```python
from build123d import *

# Parameters (mm, degrees)
BOSS_EXTRUDE1_DEPTH            = 7.5
BOSS_EXTRUDE2_DEPTH            = 7.5
CUT_EXTRUDE1_DEPTH             = 5
F_3_2_3_2_DIAMETER_HOLE1_D     = 3.2
FILLET1_R                      = 2
FILLET2_R                      = 2
CUT_EXTRUDE2_REACH             = 39.378
CUT_EXTRUDE2_END_RADIUS        = 224.5
SKETCH22_R                     = 2.1
CUT_EXTRUDE2_DIRECTION_2_DEPTH = 0.9
SKETCH23_R                     = 3.5
CUT_EXTRUDE3_DEPTH             = 2.6
SKETCH24_W                     = 2.6
SKETCH24_H                     = 3.5


with BuildPart() as part:
    # Sketch1 → Boss-Extrude1 (new body)
    with BuildSketch(Plane(origin=(0, 0, 0), x_dir=(1, 0, 0), z_dir=(0, 1, 0))):
        with BuildLine():
            ThreePointArc((-207.414551525, 32.851237658), (-210, 0), (-207.414551525, -32.851237658))
            Line((-207.414551525, -32.851237658), (-217.291434931, -34.415582309))
            ThreePointArc((-217.291434931, -34.415582309), (-220, 0), (-217.291434931, 34.415582309))
            Line((-217.291434931, 34.415582309), (-207.414551525, 32.851237658))
        make_face()
        with BuildLine():
            ThreePointArc((-217.291434931, -34.415582309), (-220, 0), (-217.291434931, 34.415582309))
            Line((-217.291434931, 34.415582309), (-220.254499953, 34.884885704))
            ThreePointArc((-220.254499953, 34.884885704), (-223, 0), (-220.254499953, -34.884885704))
            Line((-220.254499953, -34.884885704), (-217.291434931, -34.415582309))
        make_face()
        with BuildLine():
            Line((-202.969953992, 32.147282566), (-207.414551525, 32.851237658))
            ThreePointArc((-207.414551525, 32.851237658), (-210, 0), (-207.414551525, -32.851237658))
            Line((-207.414551525, -32.851237658), (-202.969953992, -32.147282566))
            ThreePointArc((-202.969953992, -32.147282566), (-205.5, 0), (-202.969953992, 32.147282566))
        make_face()
    extrude(amount=BOSS_EXTRUDE1_DEPTH)

    # Sketch19 → Boss-Extrude2 (add)
    with BuildSketch(Plane(origin=(0, 0, 0), x_dir=(1, 0, 0), z_dir=(0, 1, 0))):
        with BuildLine():
            Line((-224.019328267, 14.683002512), (-222.522539882, 14.584897818))
            ThreePointArc((-222.522539882, 14.584897818), (-223, 0), (-222.522539882, -14.584897818))
            Line((-222.522539882, -14.584897818), (-224.019328267, -14.683002512))
            ThreePointArc((-224.019328267, -14.683002512), (-224.5, 0), (-224.019328267, 14.683002512))
        make_face()
    extrude(amount=BOSS_EXTRUDE2_DEPTH)

    # Sketch15 → Cut-Extrude1 (cut)
    with BuildSketch(Plane(origin=(0, 7.5, 0), x_dir=(1, 0, 0), z_dir=(0, 1, 0))):
        with BuildLine():
            Line((-219.772609758, 10), (-209.761769634, 10))
            ThreePointArc((-209.761769634, 10), (-208.900850883, 21.457737542), (-207.414551525, 32.851237658))
            Line((-207.414551525, 32.851237658), (-217.291434931, 34.415582309))
            ThreePointArc((-217.291434931, 34.415582309), (-218.872736893, 22.242415451), (-219.772609758, 10))
        make_face()
        with BuildLine():
            ThreePointArc((-207.414551525, -32.851237658), (-208.900850883, -21.457737542), (-209.761769634, -10))
            Line((-209.761769634, -10), (-219.772609758, -10))
            ThreePointArc((-219.772609758, -10), (-218.872736893, -22.242415451), (-217.291434931, -34.415582309))
            Line((-217.291434931, -34.415582309), (-207.414551525, -32.851237658))
        make_face()
    extrude(amount=-CUT_EXTRUDE1_DEPTH, mode=Mode.SUBTRACT)

    # Ø3.2 (3.2) Diameter Hole1 (through all)
    with Locations(Plane(origin=(0, 0, 0), x_dir=(-1, 0, 0), z_dir=(0, -1, 0))):
        with Locations((214.18186009, -18.738484691), (214.18186009, 18.738484691)):
            Hole(F_3_2_3_2_DIAMETER_HOLE1_D / 2)

    # Fillet1
    fillet1_edges = [part.edges().sort_by_distance(p)[0] for p in [
        (-220.254499953, 3.75, 34.884885704),
        (-220.254499953, 3.75, -34.884885704),
        (-202.969953992, 3.75, -32.147282566),
        (-202.969953992, 3.75, 32.147282566),
    ]]
    fillet(fillet1_edges, radius=FILLET1_R)

    # Fillet2
    # the kernel refuses this fillet: 2 mm, written as the material it adds along each edge
    with BuildSketch(Plane(origin=(-222.522539882, 0, -14.584897818), x_dir=(0.06970140258603677, 0, -0.9975678996827931), z_dir=(0, 1, 0))) as fillet2_piece_1:
        with BuildLine():
            CenterArc((1.930030715, 1.99998144), FILLET2_R, 194.477374901, 75.275788142)
            Line((-0.006462156, 1.49998608), (-0.045192014, 1.489986173))
            ThreePointArc((-0.045192014, 1.489986173), (-0.043230707, 0.749820716), (-0.039999629, -0.000172324))
            Line((-0.039999629, -0.000172324), (0.000172324, -0.039999629))
            ThreePointArc((0.000172324, -0.039999629), (0.960707253, -0.037930577), (1.921242182, -0.039999629))
            Line((1.921242182, -0.039999629), (1.921414506, 0))
        make_face()
    extrude(amount=7.5)
    with BuildSketch(Plane(origin=(-222.522539882, 0, 14.584897818), x_dir=(-0.9978589232386029, 0, 0.06540312923015226), z_dir=(0, 1, 0))) as fillet2_piece_2:
        with BuildLine():
            CenterArc((1.991648107, 1.938628933), FILLET2_R, 180.493673912, 75.275788142)
            Line((-0.008277654, 1.921396676), (-0.048276169, 1.92105203))
            ThreePointArc((-0.048276169, 1.92105203), (-0.042069052, 0.960534929), (-0.04, 0))
            Line((-0.04, 0), (0, -0.04))
            ThreePointArc((0, -0.04), (0.75, -0.04), (1.490167038, -0.038772579))
            Line((1.490167038, -0.038772579), (1.5, 0))
        make_face()
    extrude(amount=7.5)

    # Cut-Extrude2: up to this cylinder (the profile starts inside it)
    cut_extrude2_end = Plane(origin=(0, 7.5, 0), z_dir=(0, -1, 0)) * Cylinder(CUT_EXTRUDE2_END_RADIUS, 528.756, mode=Mode.PRIVATE)
    # Sketch22 → Cut-Extrude2 (cut, up to the surface)
    with BuildSketch(Plane(origin=(-212.5, 0, 0), x_dir=(0, 0, -1), z_dir=(1, 0, 0)), mode=Mode.PRIVATE) as cut_extrude2_sk1:
        with Locations((0, 7.5)):
            Circle(SKETCH22_R)
    cut_extrude2_tool1 = extrude(cut_extrude2_sk1.sketch, amount=-CUT_EXTRUDE2_REACH, mode=Mode.PRIVATE) & cut_extrude2_end
    add(cut_extrude2_tool1.solids().sort_by_distance((-212.5, 7.5, 0))[0], mode=Mode.SUBTRACT)

    # Sketch22 → Cut-Extrude2 direction 2 (cut)
    with BuildSketch(Plane(origin=(-212.5, 0, 0), x_dir=(0, 0, -1), z_dir=(1, 0, 0))):
        with Locations((0, 7.5)):
            Circle(SKETCH22_R)
    extrude(amount=CUT_EXTRUDE2_DIRECTION_2_DEPTH, mode=Mode.SUBTRACT)

    # Sketch23 → Cut-Extrude3 (cut)
    with BuildSketch(Plane.ZY.offset(211.6)):
        with Locations((0, 7.439199918)):
            Circle(SKETCH23_R)
    extrude(amount=CUT_EXTRUDE3_DEPTH, mode=Mode.SUBTRACT)

    # Sketch24 → Cut-Revolve1 (revolve, cut)
    with BuildSketch(Plane(origin=(0, 7.5, 0), x_dir=(1, 0, 0), z_dir=(0, 1, 0))):
        with Locations((-223.2, 1.75)):
            Rectangle(SKETCH24_W, SKETCH24_H)
    revolve(axis=Axis((-224.5, 7.5, 0), (1, 0, 0)), mode=Mode.SUBTRACT)


solid = part.part
```
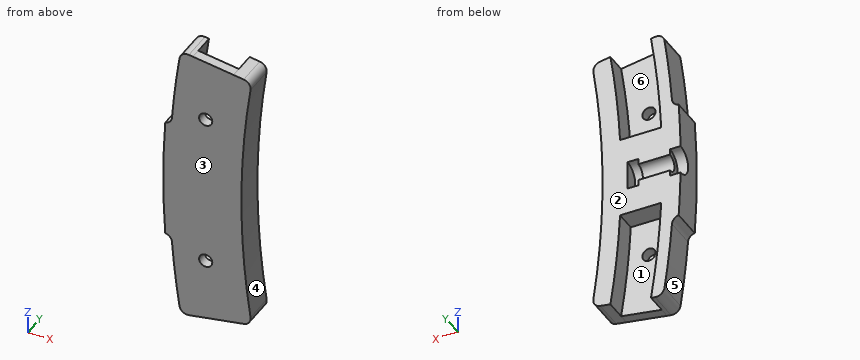
Geometry check sheet. Reference: the model listing, model coordinates, mm. Face numbers are marked on the shaded views. A direction names the side the tool comes from. Round coordinates to 2 decimals unless told otherwise and drop trailing zeros. Order: outer loops, then holes, each group sorted by start corner. A loop starts at its lowest first (then second) coordinate and runs counter-clockwise, first axis right, second up. Notation, with made-up numbers: (42, 42) - (76, 42) arc R26 ccw to (76, 72) - close; hole circle Ø11 at (-17, 25.5). An arc over 180 degrees is marked (long way). Use a Markdown table: item, result. Add a question column.
1) Section check A-A (z = 0). Record the cut outline in (x, y).
2) Section check C-C (y = 0.75). Record the cut outline in (x, z).
3) Section check D-D (z = -24). Record the cut outline in (x, y).
4) Thickness scan on line 1 along X through (y, z) = (3, 17.5); line 2 along X through (y, z) = (7.25, 26); line 3 along Z through (x, y) = (-214.25, 4.75). Record the ranges inside material, lowest first.
5) Set-up check for the marked faces 1 and 2: record each of +Z, -Z, +X, -X, +Y, -Y from which the full face is reachable in a straight line by a thin tool's end or side.
6) Mould release check, pull along X, two halves, no side actions. Record for the marked faces 3, 4, 5 and 6: released by +X, released by -X, zero draft, split by the parting line, or undercut.
7) Gauge pin test, flat ends, axial feed: P1, Ø4, axis at y = 2.5, z = 23.5, coming from the -X side; P2, Ø3, axis at y = 5.5, z = 1, coming from the +X side; P3, Ø3, axis at y = 6, z = 23.5, coming from the -X side; P4, Ø1.9, axis at x = -214.18, z = 18.74, coming from the +Y side. Record the tip position at first contact, or that the pin passes through.
Established:
| question | item | result |
|---|---|---|
| 1 | outline | (-224.5, 0) - (-205.5, 0) - (-205.5, 7.5) - (-211.6, 7.5) - (-211.6, 3.94) - (-214.2, 3.94) - (-214.2, 5.4) - (-221.9, 5.4) - (-221.9, 4) - (-224.5, 4) - close |
| 2 | outline | (-224.02, -14.68) arc R2 cw to (-222.39, -16.5) arc R223 ccw to (-220.56, -32.89) arc R2 ccw to (-218.27, -34.57) - (-204.94, -32.46) arc R2 ccw to (-203.27, -30.19) arc R205.5 cw to (-203.27, 30.19) arc R2 ccw to (-204.94, 32.46) - (-218.27, 34.57) arc R2 ccw to (-220.56, 32.89) arc R223 ccw to (-222.39, 16.5) arc R2 cw to (-224.02, 14.68) arc R224.5 ccw to start; hole circle Ø3.2 at (-214.18, -18.74); hole circle Ø3.2 at (-214.18, 18.74) |
| 3 | outline | (-221.7, 0) - (-204.09, 0) - (-204.09, 7.5) - (-208.62, 7.5) - (-208.62, 2.5) - (-218.69, 2.5) - (-218.69, 7.5) - (-221.7, 7.5) - close |
| 4 | line 1 | -222.31 to -219.3, -209.27 to -204.75 |
| 4 | line 2 | -221.48 to -218.46, -208.38 to -203.85 |
| 4 | line 3 | -10 to 10 |
| 5 | face 1 | +Y |
| 5 | face 2 | +Z, -Z, +X, -X, +Y |
| 6 | face 3 | zero draft |
| 6 | face 4 | released by +X |
| 6 | face 5 | released by -X |
| 6 | face 6 | undercut |
| 7 | P1 | x = -221.96 |
| 7 | P2 | x = -205.48 |
| 7 | P3 | x = -221.91 |
| 7 | P4 | through |
